Work out the finished part from the listing and answer in its coordinate system (mm). Face numbers are marked on the shaded views. A direction names the side the tool comes from. Coordinates: 2 decimals unless noted, no trailing zeros. Loops run counter-clockwise (first coordinate to the right, second up) from the corner with the lowest first, then second, coordinate; pieces in that order, holes last. Notation, with made-up numbers: (-7.75, 37) -> (-2.75, 37) arc R9 ccw to (-2.75, 47) -> close; hole circle Ø6 at (89.25, 65.25). An arc over 180 degrees is marked (long way). One line per question, with ' | ' between items.
```python
from build123d import *

# Parameters (mm, degrees)
F1_DEPTH = 25
F4_DEPTH = 25
F5_DEPTH = 5
F6_R     = 5
F7_R     = 10


with BuildPart() as f1:
    # F0 (on Top) → F1 (new body)
    with BuildSketch(Plane.XY):
        Polygon((60, 106.5), (-100, 106.5), (-100, -65.9319981933), (-60, -106.5), (100, -106.5), (100, 66.5), align=None)
        with BuildLine():
            Line((81, -37.5), (55, -37.5))
            ThreePointArc((55, -37.5), (38.0294372515, -44.5294372515), (31, -61.5))
            Line((31, -61.5), (31, -87.5))
            ThreePointArc((31, -87.5), (28.0710678119, -94.5710678119), (21, -97.5))
            Line((21, -97.5), (-36, -97.5))
            ThreePointArc((-36, -97.5), (-43.0710678119, -94.5710678119), (-46, -87.5))
            Line((-46, -87.5), (-46, -50.2086650483))
            ThreePointArc((-46, -50.2086650483), (-44.0202162123, -44.2357150312), (-38.8647736185, -40.6277949357))
            ThreePointArc((-38.8647736185, -40.6277949357), (6.8505042274, -13.3505042274), (34.1277949357, 32.3647736185))
            ThreePointArc((34.1277949357, 32.3647736185), (37.7357150312, 37.5202162123), (43.7086650483, 39.5))
            Line((43.7086650483, 39.5), (81, 39.5))
            ThreePointArc((81, 39.5), (88.0710678119, 36.5710678119), (91, 29.5))
            Line((91, 29.5), (91, -27.5))
            ThreePointArc((91, -27.5), (88.0710678119, -34.5710678119), (81, -37.5))
        make_face(mode=Mode.SUBTRACT)
    extrude(amount=F1_DEPTH)

    # F3 (on offset) → F4 (join)
    with BuildSketch(Plane(origin=(0, 0, 25), x_dir=(1, 0, 0), z_dir=(0, 0, -1))):
        with BuildLine():
            Line((12.1408432435, -49.3565721142), (-55.4461455939, 18.2180655315))
            ThreePointArc((-55.4461455939, 18.2180655315), (-84.1408590322, 18.6434121001), (-83.720692703, -10.0513776581))
            Line((-83.720692703, -10.0513776581), (-16.1434121001, -77.6408590322))
            ThreePointArc((-16.1434121001, -77.6408590322), (12.1408595897, -77.6434115426), (12.1434109852, -49.3591398528))
            ThreePointArc((12.1434109852, -49.3591398528), (12.1421271726, -49.3578559252), (12.1408432435, -49.3565721142))
        make_face()
        with BuildLine():
            ThreePointArc((-76.6428401008, -2.9748026994), (-77.0704295161, 11.57170605), (-62.5239981961, 11.1414905727))
            Line((-62.5239981961, 11.1414905727), (5.0697784915, -56.4276431028))
            ThreePointArc((5.0697784915, -56.4276431028), (5.0710717587, -70.5710638651), (-9.072349005, -70.5697863865))
            Line((-9.072349005, -70.5697863865), (-76.6428401008, -2.9748026994))
        make_face(mode=Mode.SUBTRACT)
    extrude(amount=-F4_DEPTH)

    # F0 (on Top) → F5 (join)
    with BuildSketch(Plane.XY):
        with BuildLine():
            ThreePointArc((31, -61.5), (38.0294372515, -44.5294372515), (55, -37.5))
            Line((55, -37.5), (81, -37.5))
            ThreePointArc((81, -37.5), (88.0710678119, -34.5710678119), (91, -27.5))
            Line((91, -27.5), (91, 29.5))
            ThreePointArc((91, 29.5), (88.0710678119, 36.5710678119), (81, 39.5))
            Line((81, 39.5), (43.7086650483, 39.5))
            ThreePointArc((43.7086650483, 39.5), (37.7357150312, 37.5202162123), (34.1277949357, 32.3647736185))
            ThreePointArc((34.1277949357, 32.3647736185), (6.8505042274, -13.3505042274), (-38.8647736185, -40.6277949357))
            ThreePointArc((-38.8647736185, -40.6277949357), (-44.0202162123, -44.2357150312), (-46, -50.2086650483))
            Line((-46, -50.2086650483), (-46, -87.5))
            ThreePointArc((-46, -87.5), (-43.0710678119, -94.5710678119), (-36, -97.5))
            Line((-36, -97.5), (21, -97.5))
            ThreePointArc((21, -97.5), (28.0710678119, -94.5710678119), (31, -87.5))
            Line((31, -87.5), (31, -61.5))
        make_face()
    extrude(amount=F5_DEPTH)

    # F6
    f6_edges = [f1.edges().sort_by_distance(p)[0] for p in [
        (-84.140859, -18.643412, 25),
        (-21.652651, 15.569253, 25),
        (6.850504, -13.350504, 25),
        (31, -74.5, 5),
        (38.029437, -44.529437, 5),
        (68, -37.5, 5),
        (88.071068, -34.571068, 5),
        (91, 1, 5),
        (88.071068, 36.571068, 5),
        (62.354333, 39.5, 5),
        (37.735715, 37.520216, 5),
        (6.850504, -13.350504, 5),
        (-44.020216, -44.235715, 5),
        (-46, -68.854333, 5),
        (-43.071068, -94.571068, 5),
        (-7.5, -97.5, 5),
        (28.071068, -94.571068, 5),
    ]]
    fillet(f6_edges, radius=F6_R)

    # F7
    f7_edges = [f1.edges().sort_by_distance(p)[0] for p in [
        (-100, 106.5, 12.5),
        (100, -106.5, 12.5),
    ]]
    fillet(f7_edges, radius=F7_R)


solid = f1.part
```
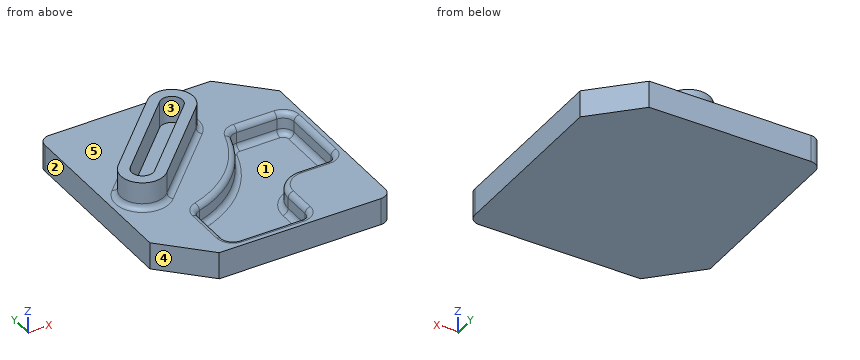
1) Find the intervals of material crossed by line 1 along Z through (x, y) = (-80, -50); line 2 along Y through (x, z) = (-37, 33.5); line 3 along Y through (x, z) = (17.5, 11), in increasing order.
Check values:
line 1: z = 0 to 25 | line 2: y = 0.22 to 14.37, 42.63 to 56.78 | line 3: y = -106.5 to -97.5, -0.97 to 106.5
2) Find section B-B (x = 66.5). Write down the section's boundary in (y, z), plus the area to 3 significant figures.
Check values:
outline: (-106.5, 0) -> (100, 0) -> (100, 25) -> (44.5, 25) arc R5 ccw to (39.5, 20) -> (39.5, 10) arc R5 cw to (34.5, 5) -> (-32.5, 5) arc R5 cw to (-37.5, 10) -> (-37.5, 20) arc R5 ccw to (-42.5, 25) -> (-106.5, 25) -> close | area: 3,620 mm^2
3) The mould has two halves that part along X. Classify the marked faces 3, 4 and 5: released by +X, released by -X, zero draft, split by the parting line, or undercut.
Check values:
face 3: undercut | face 4: released by -X | face 5: zero draft
4) For the marked faces 1 and 2, determine the directions among +Z, -Z, +X, -X, +Y, -Y from which every point of the face is accessible in a straight line to the end or side of a thin tool.
Check values:
face 1: +Z | face 2: +Z, -Z, -X, +Y, -Y
5) Flat-ended cylindrical pins translate along their axes: pin 1 (5 mm diameter, centred on x = 62, z = 12.5, fed in from +Y); pin 2 (8 mm diameter, centred on y = -76, z = 17.5, fed in from -X); pin 3 (1 mm diameter, centred on x = -3.5, z = 31, fed in from +Y) (3 decimals); pin 4 (1 mm diameter, centred on x = 16.5, y = -11, fed in from +Z). Find the tip coordinate at first contact, or state that the pin passes through.
Check values:
pin 1: stops at y = 106.5 | pin 2: stops at x = -94.02 | pin 3: stops at y = 83.475 | pin 4: stops at z = 5
